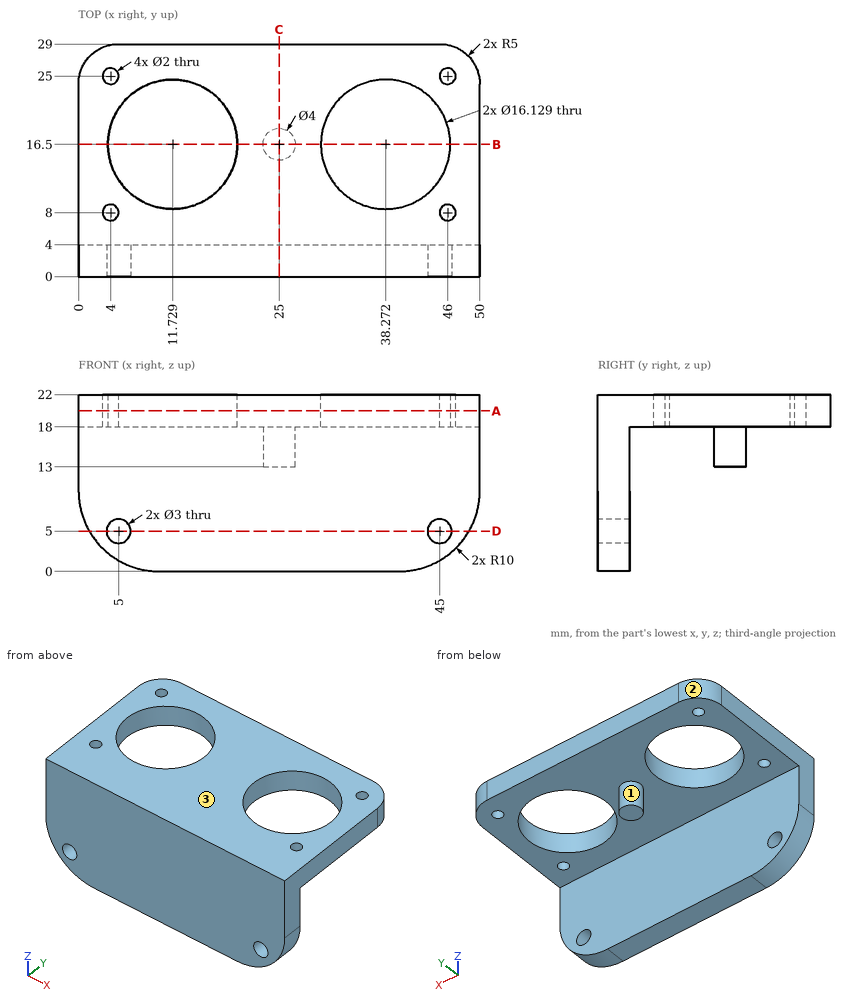
The figure shows three views and two pictorial views of one solid part (mm, origin at its lowest corner). Answer the questions. Give positions to 0.01 mm unless a question says otherwise; leave off trailing zeros. Write each loop counter-clockwise with the first axis right and the second up, starting at its lowest first coordinate (ties: lowest second). Pieces come first, ordered by that corner, then holes. Notation, with made-up numbers: (-40, 20) - (-32, 20) arc R14 cw to (-32, 26) - close; hole circle Ø9 at (30, 53). An arc over 180 degrees is marked (long way). Use one line per item in the form item = value.
1. Each of these flat-tipped pins is pushed along its axis until it touches: pin 1 Ø1.2 at (x, y) = (26, 16) entering from -Z; pin 2 Ø4 at (x, y) = (34, 8.5) entering from -Z; pin 3 Ø9 at (x, z) = (26.5, 7) entering from +Y. Where does it stop, or does it pass through?
Filled in:
pin_1 = 13
pin_2 = 18
pin_3 = 4
2. Consider L1, parallel to Y at x = 7, z = 1.25; L2, parallel to X at y = 25.25, z = 20; L3, parallel to Y at x = 23.5, z = 14.5 (1 decimal). Determine where each line is inside the solid, lowest interval first.
Filled in:
L1 = 0 to 4
L2 = 0.16 to 3.03, 4.97 to 45.03, 46.97 to 49.84
L3 = 0 to 4, 15.2 to 17.8
3. A cutting plane is placed at B-B (y = 16.5). Write down the section's boundary in (x, z) (1 decimal).
Filled in:
outline = (0, 18) - (3.7, 18) - (3.7, 22) - (0, 22) - close; (19.8, 18) - (23, 18) - (23, 13) - (27, 13) - (27, 18) - (30.2, 18) - (30.2, 22) - (19.8, 22) - close; (46.3, 18) - (50, 18) - (50, 22) - (46.3, 22) - close
4. A cutting plane is placed at A-A (z = 20). Write down the section's boundary in (x, y) (1 decimal), and give its area (3 significant figures).
Filled in:
outline = (0, 0) - (50, 0) - (50, 24) arc R5 ccw to (45, 29) - (5, 29) arc R5 ccw to (0, 24) - close; hole circle Ø2 at (4, 8); hole circle Ø2 at (4, 25); hole circle Ø16.1 at (11.7, 16.5); hole circle Ø16.1 at (38.3, 16.5); hole circle Ø2 at (46, 8); hole circle Ø2 at (46, 25)
area = 1,020 mm^2
5. A cutting plane is placed at D-D (z = 5). Write down the section's boundary in (x, y), and give its area (3 significant figures).
Filled in:
outline = (1.34, 0) - (3.5, 0) - (3.5, 4) - (1.34, 4) - close; (6.5, 0) - (43.5, 0) - (43.5, 4) - (6.5, 4) - close; (46.5, 0) - (48.66, 0) - (48.66, 4) - (46.5, 4) - close
area = 165 mm^2
6. Determine the mould class of the marked faces 1, 2 and 3 for opening direction Y: released by +Y, released by -Y, zero draft, split by the parting line, or undercut.
Filled in:
face_1 = undercut
face_2 = released by +Y
face_3 = zero draft
7. A cutting plane is placed at C-C (x = 25). Write down the section's boundary in (y, z).
Filled in:
outline = (0, 0) - (4, 0) - (4, 18) - (14.5, 18) - (14.5, 13) - (18.5, 13) - (18.5, 18) - (29, 18) - (29, 22) - (0, 22) - close
